Geometry check sheet. Reference: the model listing, model coordinates, mm. Face numbers are marked on the shaded views. A direction names the side the tool comes from. Give positions to 0.01 mm unless a question says otherwise; leave off trailing zeros. Order: outer loops, then holes, each group sorted by start corner. A loop starts at its lowest first (then second) coordinate and runs counter-clockwise, first axis right, second up. Notation, with made-up numbers: M 56.5,45.25 L 100.5,45.25 A19 cw 100.5,52.25 Z; hole C 70,-29 d11. An arc over 180 degrees is marked long. Answer as CSV lines item,"result". Start each with the question number.
Q1. Section check D-D, the plane y = -80. Record the boundary of the cut face in (x, z), then the cut area to 3 significant figures.
Q2. Thickness scan on line 1 (Y direction, x = 25, z = -17.5); line 2 (Z direction, x = 17, y = -69); line 3 (X direction, y = -46, z = -18.5). Record the ranges inside material, lowest first.
Q3. Section check A-A, the plane z = 22. Record the boundary of the cut face in (x, y).
Q4. Set-up check for the marked faces 1, 2, 3, 4 and 5: record each of +Z, -Z, +X, -X, +Y, -Y from which the full face is reachable in a straight line by a thin tool's end or side.
Q5. Section check C-C, the plane x = 1.5. Record the boundary of the cut face in (y, z), then the cut area to 3 significant figures.
Q6. Go/stop test with flat-tipped pins: pin 1 (12 mm diameter, centred on x = 14, z = -13, fed in from -Y); pin 2 (1 mm diameter, centred on x = 21.5, z = 14, fed in from -Y); pin 3 (10.5 mm diameter, centred on x = 3.5, z = 6.5, fed in from +Y). Record where each tip stops, or that it passes through.
Q7. Section check B-B, the plane z = 8.5. Record the boundary of the cut face in (x, y), then the cut area to 3 significant figures.
```python
from build123d import *

# Parameters (mm, degrees)
F0_W      = 60
F0_H      = 50
F1_DEPTH  = 30
F2_W      = 25
F2_H      = 10
F3_DEPTH  = 30.001
F5_DEPTH  = 40.001
F6_DEPTH  = 10.001
F9_DEPTH  = 30
F11_DEPTH = 30.001


with BuildPart() as f1:
    # F0 (on Front) → F1 (new body)
    with BuildSketch(Plane.XZ):
        Rectangle(F0_W, F0_H)
    extrude(amount=F1_DEPTH)

    # F2 (on face) → F3 (cut, through all)
    with BuildSketch(Plane.XZ.offset(30)):
        with Locations((0, 20)):
            Rectangle(F2_W, F2_H)
    extrude(amount=-F3_DEPTH, mode=Mode.SUBTRACT)

    # F4 (on face) → F5 (cut, through all)
    with BuildSketch(Plane.XY.offset(15)):
        Polygon((-17.5, -10), (-12.5, -10), (17.5, -10), (17.5, 0), (-17.5, 0), align=None)
    extrude(amount=-F5_DEPTH, mode=Mode.SUBTRACT)

    # F6 (cut, through all): faces of the model
    f6_faces = [f1.faces().sort_by_distance(p)[0] for p in [
        (15, -5, 15),
        (-15, -5, 15),
    ]]
    extrude(f6_faces, amount=-F6_DEPTH, mode=Mode.SUBTRACT)

    # F8 (on offset) → F9 (join)
    with BuildSketch(Plane.XY.offset(5)):
        Polygon((20.0490429997, -29.9998670816), (-20.0000924617, -29.9999825656), (-20.0000924617, -119.9999825656), (19.9999075383, -119.9999825656), align=None)
    extrude(amount=-F9_DEPTH)

    # F10 (on face) → F11 (cut, through all)
    with BuildSketch(Plane.XY.offset(5)):
        Polygon((20.0136015809, -94.9169696898), (-9.24617e-05, -119.9999825656), (19.9999075383, -119.9999825656), align=None)
        Polygon((-9.24617e-05, -119.9999825656), (-20.0000924617, -93.8219279051), (-20.0000924617, -119.9999825656), align=None)
    extrude(amount=-F11_DEPTH, mode=Mode.SUBTRACT)


solid = f1.part
```
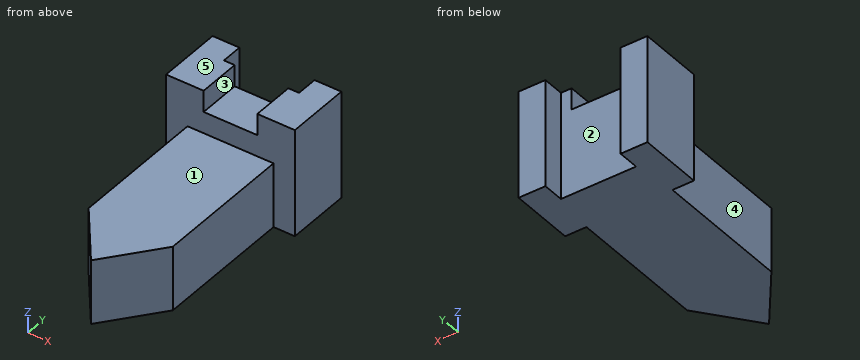
Answer block:
1,outline,"M -20,-25 L 20.02,-25 L 20.02,5 L -20,5 Z"
1,area,"1,200 mm2"
2,line 1,"y = -30 to 0"
2,line 2,"z = -25 to 5"
2,line 3,"x = -20 to 20.04"
3,outline,"M -30,-30 L -12.5,-30 L -12.5,-10 L -17.5,-10 L -17.5,0 L -30,0 Z; M 12.5,-30 L 30,-30 L 30,0 L 17.5,0 L 17.5,-10 L 12.5,-10 Z"
4,face 1,"+Z, +X, -X, -Y"
4,face 2,"+Z, -Z, +Y"
4,face 3,"+Z, +Y, -Y"
4,face 4,"+Z, -Z, -X, -Y"
4,face 5,"+Z, +X, -X, +Y, -Y"
5,outline,"M -118.12,-25 L -10,-25 L -10,15 L -30,15 L -30,5 L -118.12,5 Z"
5,area,"3,440 mm2"
6,pin 1,"stops at y = -109.97"
6,pin 2,"stops at y = -30"
6,pin 3,"stops at y = -10"
7,outline,"M -30,-30 L 30,-30 L 30,0 L 17.5,0 L 17.5,-10 L -17.5,-10 L -17.5,0 L -30,0 Z"
7,area,"1,450 mm2"
